CAD build for the part. Positions are in the model's coordinates, mm. Coordinates: 2 decimals unless noted, no trailing zeros. Order: outer loops, then holes, each group sorted by start corner. A loop starts at its lowest first (then second) coordinate and runs counter-clockwise, first axis right, second up. Notation, with made-up numbers: M 35,49.5 L 39,49.5 A25 ccw 39,62.5 Z; hole C -10,55 d8. An arc over 180 degrees is marked long. One line per item, written item: value.
from build123d import *

# Parameters (mm, degrees)
SKETCH1_W           = 473.075
SKETCH1_H           = 95.25
BOSS_EXTRUDE1_DEPTH = 3.175
SKETCH3_W           = 78.74
SKETCH3_H           = 51.308
CUT_EXTRUDE2_DEPTH  = 242.305221983
SKETCH4_R           = 8.255
CUT_EXTRUDE3_DEPTH  = 242.305221983
SKETCH5_R           = 1.5875
CUT_EXTRUDE4_DEPTH  = 242.305221983
SKETCH6_W           = 3.175
SKETCH6_H           = 95.25
BOSS_EXTRUDE2_DEPTH = 377.825
SKETCH7_R           = 3.81
SKETCH7_W           = 50.8
SKETCH7_H           = 73.025
CUT_EXTRUDE5_DEPTH  = 381
CUT_EXTRUDE6_DEPTH  = 381


with BuildPart() as part:
    # Sketch1 → Boss-Extrude1 (new body)
    with BuildSketch(Plane.XY):
        Rectangle(SKETCH1_W, SKETCH1_H)
    extrude(amount=BOSS_EXTRUDE1_DEPTH)

    # Sketch3 → Cut-Extrude2 (cut, through all)
    with BuildSketch(Plane.XY.offset(3.175)):
        with Locations((0, 6.731)):
            Rectangle(SKETCH3_W, SKETCH3_H)
    extrude(amount=-CUT_EXTRUDE2_DEPTH, mode=Mode.SUBTRACT)

    # Sketch4 → Cut-Extrude3 (cut, through all)
    with BuildSketch(Plane.XY.offset(3.175)):
        with Locations((37.592, -35.814)):
            Circle(SKETCH4_R)
    extrude(amount=-CUT_EXTRUDE3_DEPTH, mode=Mode.SUBTRACT)

    # Sketch5 → Cut-Extrude4 (cut, through all)
    with BuildSketch(Plane.XY.offset(3.175)):
        with Locations((-44.196, 40.259)):
            Circle(SKETCH5_R)
        with Locations((44.196, 40.259)):
            Circle(SKETCH5_R)
        with Locations((-44.196, -24.765)):
            Circle(SKETCH5_R)
        with Locations((44.196, -24.765)):
            Circle(SKETCH5_R)
    extrude(amount=-CUT_EXTRUDE4_DEPTH, mode=Mode.SUBTRACT)

    # Sketch6 → Boss-Extrude2 (add)
    with BuildSketch(Plane(origin=(0, 0, 0), x_dir=(-1, 0, 0), z_dir=(0, 0, -1))):
        with Locations((234.95, 0)):
            Rectangle(SKETCH6_W, SKETCH6_H)
    extrude(amount=BOSS_EXTRUDE2_DEPTH)

    # Sketch7 → Cut-Extrude5 (cut)
    with BuildSketch(Plane.ZY.offset(236.5375)):
        with Locations((-254.127, -28.575)):
            Circle(SKETCH7_R)
        with Locations((-314.325, -7.9375)):
            Rectangle(SKETCH7_W, SKETCH7_H)
    extrude(amount=-CUT_EXTRUDE5_DEPTH, mode=Mode.SUBTRACT)

    # Sketch8 → Cut-Extrude6 (cut)
    with BuildSketch(Plane.XY.offset(3.175)):
        with BuildLine():
            Line((88.9, 31.75), (215.9, 31.75))
            ThreePointArc((215.9, 31.75), (219.71, 27.94), (215.9, 24.13))
            Line((215.9, 24.13), (88.9, 24.13))
            ThreePointArc((88.9, 24.13), (85.09, 27.94), (88.9, 31.75))
        make_face()
        with BuildLine():
            Line((88.9, 12.563594852), (215.9, 12.563594852))
            ThreePointArc((215.9, 12.563594852), (219.71, 8.753594852), (215.9, 4.943594852))
            Line((215.9, 4.943594852), (88.9, 4.943594852))
            ThreePointArc((88.9, 4.943594852), (85.09, 8.753594852), (88.9, 12.563594852))
        make_face()
        with BuildLine():
            Line((88.9, -6.256272006), (215.9, -6.256272006))
            ThreePointArc((215.9, -6.256272006), (219.71, -10.066272006), (215.9, -13.876272006))
            Line((215.9, -13.876272006), (88.9, -13.876272006))
            ThreePointArc((88.9, -13.876272006), (85.09, -10.066272006), (88.9, -6.256272006))
        make_face()
        with BuildLine():
            Line((88.9, -24.84600572), (215.9, -24.84600572))
            ThreePointArc((215.9, -24.84600572), (219.71, -28.65600572), (215.9, -32.46600572))
            Line((215.9, -32.46600572), (88.9, -32.46600572))
            ThreePointArc((88.9, -32.46600572), (85.09, -28.65600572), (88.9, -24.84600572))
        make_face()
        with BuildLine():
            Line((-88.9, -24.84600572), (-215.9, -24.84600572))
            ThreePointArc((-215.9, -24.84600572), (-219.71, -28.65600572), (-215.9, -32.46600572))
            Line((-215.9, -32.46600572), (-88.9, -32.46600572))
            ThreePointArc((-88.9, -32.46600572), (-85.09, -28.65600572), (-88.9, -24.84600572))
        make_face()
        with BuildLine():
            Line((-88.9, -6.256272006), (-215.9, -6.256272006))
            ThreePointArc((-215.9, -6.256272006), (-219.71, -10.066272006), (-215.9, -13.876272006))
            Line((-215.9, -13.876272006), (-88.9, -13.876272006))
            ThreePointArc((-88.9, -13.876272006), (-85.09, -10.066272006), (-88.9, -6.256272006))
        make_face()
        with BuildLine():
            Line((-88.9, 12.563594852), (-215.9, 12.563594852))
            ThreePointArc((-215.9, 12.563594852), (-219.71, 8.753594852), (-215.9, 4.943594852))
            Line((-215.9, 4.943594852), (-88.9, 4.943594852))
            ThreePointArc((-88.9, 4.943594852), (-85.09, 8.753594852), (-88.9, 12.563594852))
        make_face()
        with BuildLine():
            Line((-88.9, 31.75), (-215.9, 31.75))
            ThreePointArc((-215.9, 31.75), (-219.71, 27.94), (-215.9, 24.13))
            Line((-215.9, 24.13), (-88.9, 24.13))
            ThreePointArc((-88.9, 24.13), (-85.09, 27.94), (-88.9, 31.75))
        make_face()
    extrude(amount=-CUT_EXTRUDE6_DEPTH, mode=Mode.SUBTRACT)


solid = part.part
Q1. Slice it at B-B (z = -277). List the corners of the cut face in (x, y) (1 decimal), plus the area to 3 significant figures.
Recorded:
outline: M -236.5,-47.6 L -233.4,-47.6 L -233.4,47.6 L -236.5,47.6 Z
area: 302 mm^2
Q2. Slice it at A-A (x = 142). List the corners of the cut face in (y, z) (3 decimals).
Recorded:
outline: M -47.625,0 L -32.466,0 L -32.466,3.175 L -47.625,3.175 Z; M -24.846,0 L -13.876,0 L -13.876,3.175 L -24.846,3.175 Z; M -6.256,0 L 4.944,0 L 4.944,3.175 L -6.256,3.175 Z; M 12.564,0 L 24.13,0 L 24.13,3.175 L 12.564,3.175 Z; M 31.75,0 L 47.625,0 L 47.625,3.175 L 31.75,3.175 Z
Q3. Mould opens along X. For faces 1 (the face through (36.52, -27.63, 1.61)), 2 (the face through (-233.362, -1, -186)), 3 (the face through (-236.538, -1, -185)), 4 (the face through (-2, -20, 0)) say: released by +X, released by -X, zero draft, split by the parting line, or undercut.
Recorded:
face 1: undercut
face 2: released by +X
face 3: released by -X
face 4: zero draft
Q4. Pin check, flat tip, straight feed: pin 1 Ø10 at (x, y) = (111.5, -15.5) entering from -Z. Stop position of the tip, or through.
Recorded:
pin 1: stops at z = 0
Q5. Slice it at C-C (x = -72). List the corners of the cut face in (y, z) (3 decimals).
Recorded:
outline: M -47.625,0 L 47.625,0 L 47.625,3.175 L -47.625,3.175 Z
Q6. Drill centre lines: line 1 along Z through (x, y) = (206.5, 0.5) (3 decimals); line 2 along X through (y, z) = (-43, -82.5). Where is each one in solid material? Low to high.
Recorded:
line 1: z = 0 to 3.175
line 2: x = -236.54 to -233.36
